Check sheet for the drawn part. Datum: minimum x, y, z corner. Units: mm. A direction names the side the tool comes from. Give positions to 0.01 mm unless a question says otherwise; leave off trailing zeros. Write each loop counter-clockwise with the first axis right and the second up, starting at its lowest first coordinate (ties: lowest second). Pieces come first, ordered by that corner, then holes. Notation, with made-up numbers: M -32,32.25 L 24,32.25 A37 cw 24,70.25 Z; hole C 9.5,37.25 d6. An arc over 180 degrees is marked long. Use CSV: the item, a comma, the result in double quotes. Start each with the question number.
1. Scan lines: line 1 (X direction, y = 17, z = 53) (1 decimal); line 2 (Z direction, x = 120, y = 86) (1 decimal); line 3 (Y direction, x = 105, z = 70). Record each from-to range of solid material in increasing order.
2. Cross-section at B-B, the plane x = 121.5. State how many separate pieces and enclosed holes the cut face has, and give its area (3 significant figures).
3. Mould release check, pull along X, two halves, no side actions. Record for the marked faces 3, 4, 5 and 6: +X half, -X half, draft (parallel to the pull), parting line (faces both ways), or undercut.
4. Cross-section at A-A, the plane y = 86.25. Enter the section's corners in (x, z) (1 decimal).
5. Access from +Z, -Z, +X, -X, +Y, -Y to the whole of each face (thin tool, end or side, straight path). Record for the marked faces 1 and 2.
6. Depth check by flat-ended pin: P1, Ø1, axis at x = 86.5, z = 49, coming from the +Y side. Enter the tip coordinate at first touch or a pass-through.
7. Cross-section at D-D, the plane x = 47.5. Enter the section's corners in (y, z) (1 decimal), and give its area (3 significant figures).
8. Cross-section at C-C, the plane z = 22.5. Enter the section's corners in (x, y) (1 decimal).
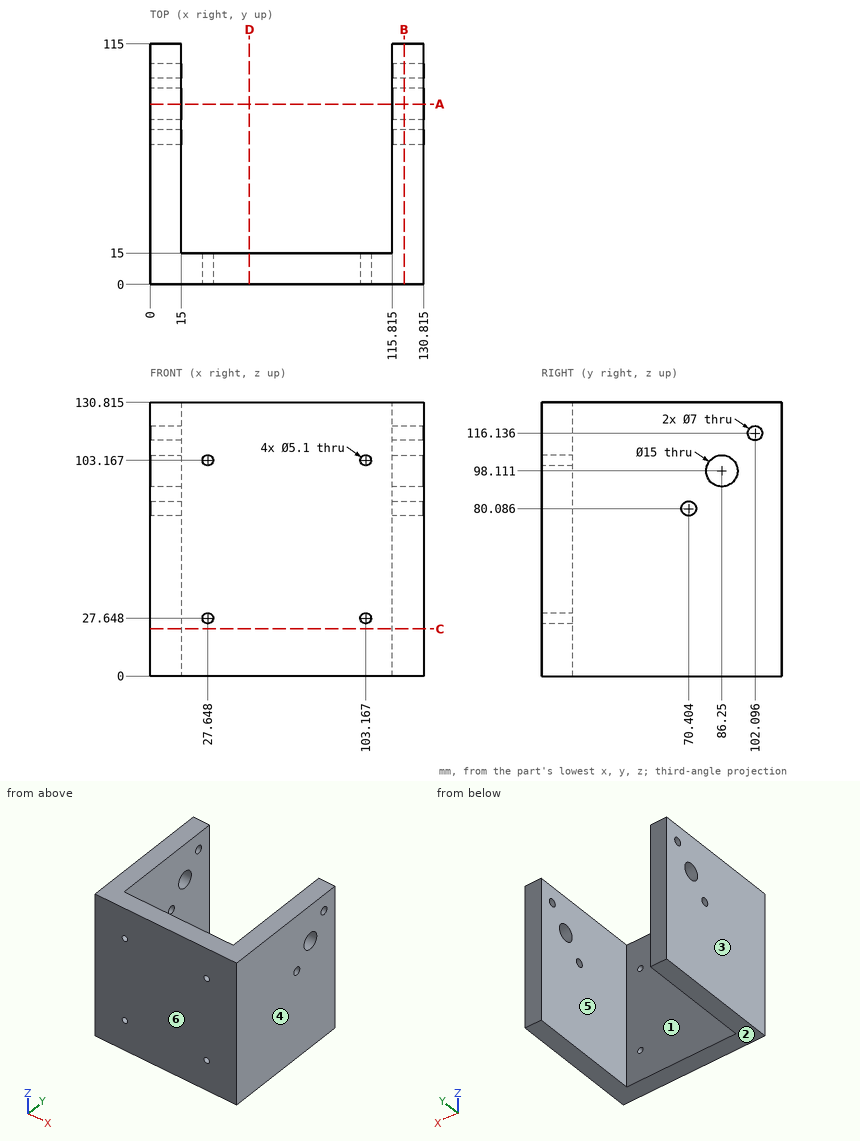
Worked answers:
1,line 1,"x = 0 to 15, 115.8 to 130.8"
1,line 2,"z = 0 to 90.6, 105.6 to 130.8"
1,line 3,"y = 0 to 15"
2,separate pieces,"1"
2,enclosed holes,"3"
2,area,"14,800 mm^2"
3,face 3,"-X half"
3,face 4,"+X half"
3,face 5,"undercut"
3,face 6,"draft"
4,outline,"M 0,0 L 15,0 L 15,90.6 L 0,90.6 Z; M 0,105.6 L 15,105.6 L 15,130.8 L 0,130.8 Z; M 115.8,0 L 130.8,0 L 130.8,90.6 L 115.8,90.6 Z; M 115.8,105.6 L 130.8,105.6 L 130.8,130.8 L 115.8,130.8 Z"
5,face 1,"+Z, -Z, +Y"
5,face 2,"-Z, +X, -X, +Y, -Y"
6,P1,"stops at y = 15"
7,outline,"M 0,0 L 15,0 L 15,130.8 L 0,130.8 Z"
7,area,"1,960 mm^2"
8,outline,"M 0,0 L 130.8,0 L 130.8,115 L 115.8,115 L 115.8,15 L 15,15 L 15,115 L 0,115 Z"
